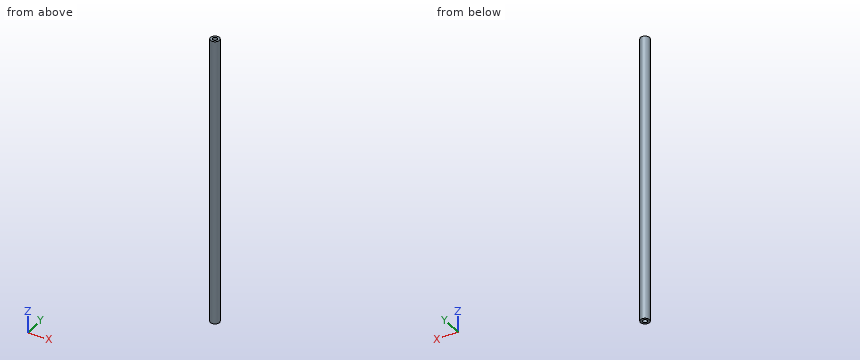
Autodesk Inventor part; units mm, degrees
ref_plane "YZ Plane" through (0, 0, 0) normal (1, 0, 0) x (0, 1, 0)
ref_plane "XZ Plane" through (0, 0, 0) normal (0, 1, 0) x (-1, 0, 0)
ref_plane "XY Plane" through (0, 0, 0) normal (0, 0, 1) x (1, 0, 0)
sketch "Sketch1" plane through (0, 0, 0) normal (0, 0, 1) x (1, 0, 0)
  circle A0 centre (0, 0) radius 3.175
  dimension "d0" = 6.35
extrude "Extrusion1" add sketch "Sketch1" along normal mid plane 203.708
sketch "Sketch2" plane through (0, 0, 101.854) normal (0, 0, 1) x (1, 0, 0)
  point P0 (0, 0)
  point P1 (0, 0)
hole "Hole1" at (0, 0, 101.854) direction (0, 0, -1) diameter 3.302 depth 12.2936 tip angle 118
mirror "Mirror1" about plane through (0, 0, 0) normal (0, 0, 1) of "Hole1"
Verification items for the finished model (mm, model axes). Give positions to 0.01 mm unless a question says otherwise; leave off trailing zeros. Write each loop counter-clockwise with the first axis right and the second up, starting at its lowest first coordinate (ties: lowest second). Pieces come first, ordered by that corner, then holes. Notation, with made-up numbers: (58.5, -18.5) - (100.5, -18.5) arc R30 cw to (100.5, 13.5) - close; hole circle Ø5 at (82.5, 29). An arc over 180 degrees is marked (long way). Put each result on its own line as item: value.
Q1. Scan lines: probe 1 along Y at (x, z) = (0, -93.5) (3 decimals); probe 2 along Y at (x, z) = (0.25, -30); probe 3 along Z at (x, y) = (0, 0). Record each from-to range of solid material in increasing order. Write a range as from..to.
Result:
probe 1: -3.175..-1.651, 1.651..3.175
probe 2: -3.17..3.17
probe 3: -88.57..88.57
Q2. Depth check by flat-ended pin: P1, Ø3, axis at x = 1, y = 0.5, coming from the +Z side; P2, Ø2.5, axis at x = 0, y = 0, coming from the +Z side. Enter the tip coordinate at first touch or a pass-through.
Result:
P1: z = 101.85
P2: z = 89.32
Q3. Section check A-A on z = 83. Record the cut outline in (x, y) (3 decimals).
Result:
outline: circle Ø6.35 at (0, 0)
